```python
from build123d import *

# Parameters (mm, degrees)
SKETCH1_R           = 22
SKETCH1_R_2         = 8
BOSS_EXTRUDE1_DEPTH = 5
SKETCH2_R           = 14
SKETCH2_R_2         = 8
BOSS_EXTRUDE2_DEPTH = 6


with BuildPart() as part:
    # Sketch1 → Boss-Extrude1 (new body)
    with BuildSketch(Plane(origin=(0, 0, 0), x_dir=(1, 0, 0), z_dir=(0, 1, 0))):
        with Locations(Location((0, 0, 0), (0, 0, 270))):
            Circle(SKETCH1_R)
        with Locations(Location((0, 0, 0), (0, 0, 270))):
            Circle(SKETCH1_R_2, mode=Mode.SUBTRACT)
    extrude(amount=BOSS_EXTRUDE1_DEPTH)

    # Sketch2 → Boss-Extrude2 (add)
    with BuildSketch(Plane(origin=(0, 5, 0), x_dir=(1, 0, 0), z_dir=(0, 1, 0))):
        with Locations(Location((0, 0, 0), (0, 0, 270))):
            Circle(SKETCH2_R)
        with Locations(Location((0, 0, 0), (0, 0, 270))):
            Circle(SKETCH2_R_2, mode=Mode.SUBTRACT)
    extrude(amount=BOSS_EXTRUDE2_DEPTH)

    # Sketch3 → Revolve1 (revolve)
    with BuildSketch(Plane.XY, mode=Mode.PRIVATE) as revolve1_sk:
        with BuildLine():
            Line((8, 11), (11.370346923, 31.519425266))
            ThreePointArc((11.370346923, 31.519425266), (11.879606474, 32.419695227), (12.850513419, 32.776305659))
            Line((12.850513419, 32.776305659), (15.810314893, 32.776305659))
            ThreePointArc((15.810314893, 32.776305659), (16.953704462, 32.247212604), (17.29048139, 31.033186053))
            Line((17.29048139, 31.033186053), (14, 11))
            Line((14, 11), (8, 11))
        make_face()
    revolve(revolve1_sk.sketch.rotate(Axis((0, 0, 0), (0, 1, 0)), 90), axis=Axis((0, 0, 0), (0, 1, 0)))


solid = part.part
```
CAD build for the part. Positions are in the model's coordinates, mm. A direction names the side the tool comes from. Round coordinates to 2 decimals unless told otherwise and drop trailing zeros. Loops run counter-clockwise (first coordinate to the right, second up) from the corner with the lowest first, then second, coordinate; pieces in that order, holes last. Notation, with made-up numbers: M 34,53.5 L 39,53.5 A35 ccw 39,86.5 Z; hole C 38,65.5 d7. An arc over 180 degrees is marked long. Use a Markdown table: item, result. Add a question column.
(1) Cut at B-B (z = 0). Give the cut face in (x, y).
(2) Cut at C-C (y = 4). Give the cut face in (x, z), and give its area (3 significant figures).
(3) Cut at A-A (x = 0). Give the cut face in (y, z), and give its area (3 significant figures).
(4) Drill centre lines: line 1 (X direction, y = 4, z = 0); line 2 (X direction, y = 8, z = 0); line 3 (Y direction, x = 12, z = -14). Where is each one in solid material? Low to high.
(5) Flat gauge pins, fed straight in: pin 1 (2 mm diameter, centred on y = 29, z = -14, fed in from +X); pin 2 (2 mm diameter, centred on x = -9.5, z = -6.5, fed in from +Y); pin 3 (1.5 mm diameter, centred on y = 29, z = -15.5, fed in from -X); pin 4 (4 mm diameter, centred on x = 3, z = -5.5, fed in from -Y). Where does each tip first touch, or does it go through?
(6) Pull direction Z, two halves, no side cores. Call faces 3 (the face through (-4.583, 18.65, -14.552)), 4 (the face through (-13, 32.776, -1)), 5 (the face through (-7.81, 5.42, -1.73)): +Z half, -Z half, draft (parallel to the pull), parting line (faces both ways), or undercut.
(7) Cut at D-D (y = 29). Give the cut face in (x, z).
(8) Which spindle directions (+Z, -Z, +X, -X, +Y, -Y) get a long thin tool onto all of the face, cutting with end or side? Do faces 1 (the face through (-9, 0, 0)), 2 (the face through (-13.67, 7.96, -3.03)). Say none if no direction does.
Geometry says:
| question | item | result |
|---|---|---|
| 1 | outline | M -22,0 L -8,0 L -8,11 L -11.37,31.52 A1.5 ccw -12.85,32.78 L -15.81,32.78 A1.5 ccw -17.29,31.03 L -14,11 L -14,5 L -22,5 Z; M 8,0 L 22,0 L 22,5 L 14,5 L 14,11 L 17.29,31.03 A1.5 ccw 15.81,32.78 L 12.85,32.78 A1.5 ccw 11.37,31.52 L 8,11 Z |
| 2 | outline | C 0,0 d44; hole C 0,0 d16 |
| 2 | area | 1,320 mm² |
| 3 | outline | M 0,-22 L 5,-22 L 5,-14 L 11,-14 L 31.03,-17.29 A1.5 ccw 32.78,-15.81 L 32.78,-12.85 A1.5 ccw 31.52,-11.37 L 11,-8 L 0,-8 Z; M 0,8 L 11,8 L 31.52,11.37 A1.5 ccw 32.78,12.85 L 32.78,15.81 A1.5 ccw 31.03,17.29 L 11,14 L 5,14 L 5,22 L 0,22 Z |
| 3 | area | 471 mm² |
| 4 | line 1 | x = -22 to -8, 8 to 22 |
| 4 | line 2 | x = -14 to -8, 8 to 14 |
| 4 | line 3 | y = 0 to 5 |
| 5 | pin 1 | stops at x = 10.91 |
| 5 | pin 2 | stops at y = 32.74 |
| 5 | pin 3 | stops at x = -8.39 |
| 5 | pin 4 | stops at y = 0 |
| 6 | face 3 | parting line |
| 6 | face 4 | draft |
| 6 | face 5 | undercut |
| 7 | outline | C 0,0 d33.91; hole C 0,0 d21.91 |
| 8 | face 1 | +Z, -Z, +X, -X, -Y |
| 8 | face 2 | none |
